The figure shows three views and two pictorial views of one solid part (mm, origin at its lowest corner). Answer the questions. A direction names the side the tool comes from. Give positions to 0.01 mm unless a question says otherwise; leave off trailing zeros. Loops run counter-clockwise (first coordinate to the right, second up) from the corner with the lowest first, then second, coordinate; pieces in that order, holes last. Notation, with made-up numbers: (48.5, 31.25) - (102.5, 31.25) arc R17 cw to (102.5, 59.25) - close; hole circle Ø6 at (-31.75, 9). An arc over 180 degrees is marked (long way). Use a Markdown table: item, result. Add a question column.
Item 1: A cutting plane is placed at A-A (x = 14). Determine the outline of the cut face in (y, z), plus the area to 3 significant figures.
Item 2: Which of the six approach directions +Z, -Z, +X, -X, +Y, -Y give full straight-line access (tool end or side, diameter ignored) to the marked faces 1 and 2?
Item 3: Each of these flat-tipped pins is pushed along its axis until it touches: P1, Ø6, axis at y = 3, z = 3, coming from the -X side; P2, Ø12, axis at y = 12, z = 3, coming from the +X side; P3, Ø4, axis at x = 23.5, y = 17.5, coming from the +Z side. Where does it stop, or does it pass through?
Item 4: A cutting plane is placed at D-D (y = 23). Determine the outline of the cut face in (x, z).
Item 5: Consider probe 1 along Y at (x, z) = (6, 14.25); probe 2 along Y at (x, z) = (7, 25.5); probe 3 along Y at (x, z) = (7.25, 23.5). Determine where each line is inside the solid, lowest interval first. Write a range as [from, to].
Item 6: A cutting plane is placed at C-C (y = 6.75). Determine the outline of the cut face in (x, z).
Item 7: A cutting plane is placed at B-B (z = 14). Determine the outline of the cut face in (x, y), plus the area to 3 significant figures.
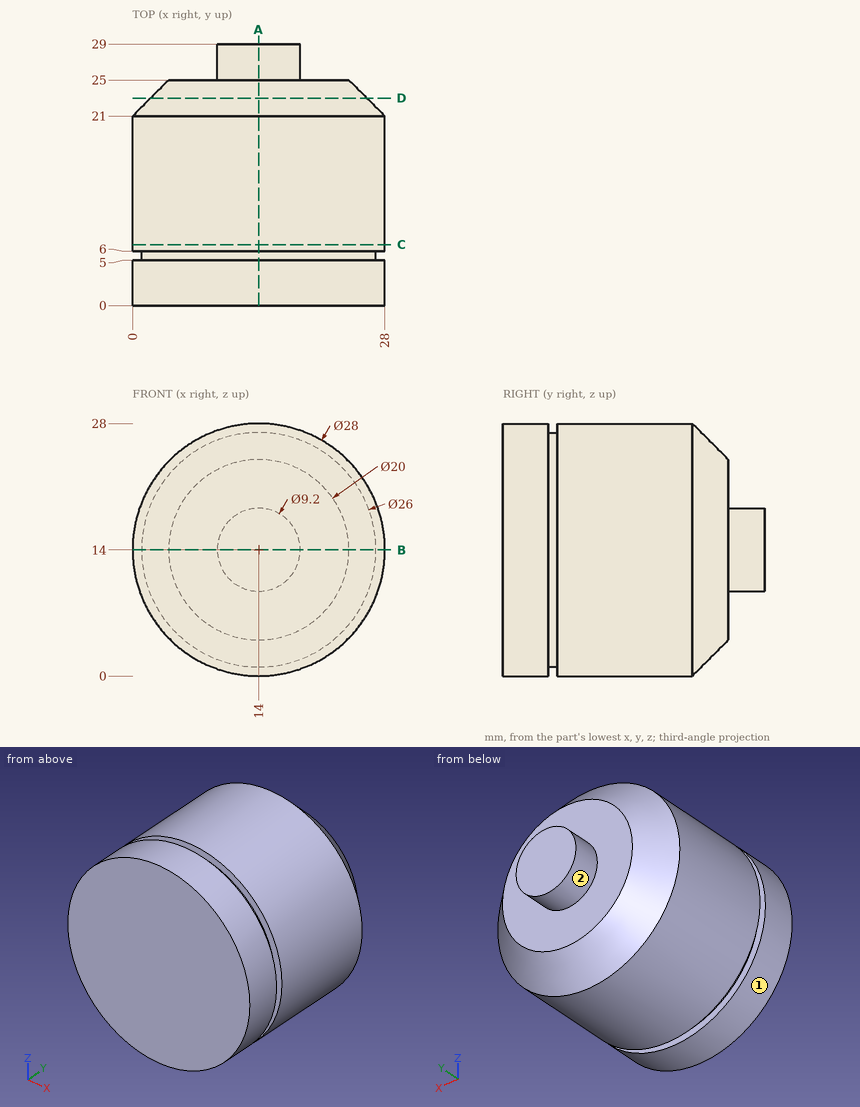
Geometry says:
| question | item | result |
|---|---|---|
| 1 | outline | (0, 0) - (5, 0) - (5, 1) - (6, 1) - (6, 0) - (21, 0) - (25, 4) - (25, 9.4) - (29, 9.4) - (29, 18.6) - (25, 18.6) - (25, 24) - (21, 28) - (6, 28) - (6, 27) - (5, 27) - (5, 28) - (0, 28) - close |
| 1 | area | 719 mm² |
| 2 | face 1 | +Y, -Y |
| 2 | face 2 | +Y |
| 3 | P1 | x = 2.51 |
| 3 | P2 | x = 27.08 |
| 3 | P3 | z = 25.82 |
| 4 | outline | circle Ø24 at (14, 14) |
| 5 | probe 1 | [0, 25] |
| 5 | probe 2 | [0, 5], [6, 21.54] |
| 5 | probe 3 | [0, 23.35] |
| 6 | outline | circle Ø28 at (14, 14) |
| 7 | outline | (0, 0) - (28, 0) - (28, 5) - (27, 5) - (27, 6) - (28, 6) - (28, 21) - (24, 25) - (18.6, 25) - (18.6, 29) - (9.4, 29) - (9.4, 25) - (4, 25) - (0, 21) - (0, 6) - (1, 6) - (1, 5) - (0, 5) - close |
| 7 | area | 719 mm² |
